Study the drawing (mm; zero at the part's minimum x, y, z) and answer. A direction names the side the tool comes from. Round coordinates to 2 decimals unless told otherwise and drop trailing zeros. Write each loop counter-clockwise with the first axis right and the second up, starting at its lowest first coordinate (ties: lowest second). Pieces come first, ordered by that corner, then holes. Notation, with made-up numbers: (19.5, -12.75) - (33.5, -12.75) arc R27 ccw to (33.5, 23.25) - close; hole circle Ø11 at (23, -26). An arc over 180 degrees is marked (long way). Use one line per item in the form item = value. Start each with the question number.
1) For a pull along Z with two mould halves and no side action, classify the marked faces 1, 2, 3 and 4 as released by +Z, released by -Z, zero draft, split by the parting line, or undercut.
2) Each of these flat-tipped pins is pushed along its axis until it touches: pin 1 (8.5 mm diameter, centred on y = 7, z = 6, fed in from +X); pin 2 (3 mm diameter, centred on x = 4.5, y = 5.5, fed in from -Z); pin 3 (3 mm diameter, centred on x = 3.5, y = 2.5, fed in from -Z); pin 4 (5 mm diameter, centred on x = 15, z = 37.5, fed in from -Y). Where does it stop, or does it pass through?
3) The part is cut by section D-D, the plane x = 15. Give the vertices of the cut face in (y, z) (3 decimals), plus the area to 3 significant figures.
4) Consider line 1 along X through (y, z) = (8.25, 12.35) (3 decimals); line 2 along Z through (x, y) = (1.25, 6.5); line 3 along Y through (x, z) = (8, 46). Determine where each line is inside the solid, lowest interval first. Write a range as from..to.
5) The part is cut by section A-A, the plane y = 7. Give the vertices of the cut face in (x, z) (3 decimals).
6) The part is cut by section B-B, the plane x = 10.25. Give the vertices of the cut face in (y, z) (3 decimals), plus the area to 3 significant figures.
7) The part is cut by section C-C, the plane z = 52. Give the vertices of the cut face in (x, y), plus the area to 3 significant figures.
8) For the marked faces 5, 6 and 7, determine the directions among +Z, -Z, +X, -X, +Y, -Y from which every point of the face is accessible in a straight line to the end or side of a thin tool.
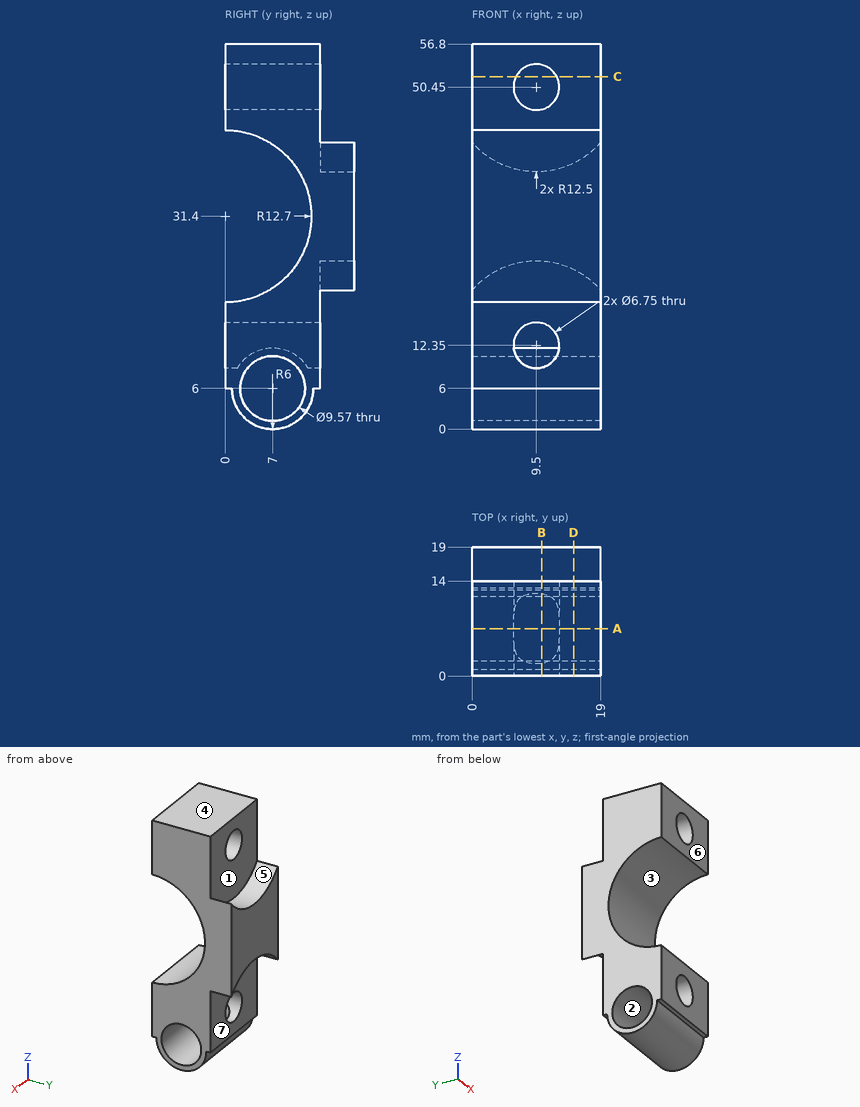
Geometry results:
q1.face_1 = zero draft
q1.face_2 = undercut
q1.face_3 = undercut
q1.face_4 = released by +Z
q2.pin_1 = through
q2.pin_2 = 0
q2.pin_3 = 0.8
q2.pin_4 = 9.35
q3.outline = (0, 6) - (1, 6) arc R6 ccw to (13, 6) - (14, 6) - (14, 23.575) - (19, 23.575) - (19, 39.225) - (14, 39.225) - (14, 56.8) - (0, 56.8) - (0, 44.1) arc R12.7 cw to (0, 18.7) - close; hole circle Ø9.57 at (7, 6)
q3.area = 521 mm2
q4.line_1 = 0..6.125, 12.875..19
q4.line_2 = 0.02..1.24, 10.76..20.49, 42.31..56.8
q4.line_3 = 0..14
q5.outline = (0, 0) - (19, 0) - (19, 1.215) - (0, 1.215) - close; (0, 10.785) - (19, 10.785) - (19, 20.803) - (0, 20.803) - close; (0, 41.997) - (19, 41.997) - (19, 56.8) - (0, 56.8) - close; hole circle Ø6.75 at (9.5, 50.45); hole (6.143, 12) - (12.857, 12) arc R3.375 ccw (long way) to start
q6.outline = (0, 6) - (1, 6) arc R6 ccw to (13, 6) - (14, 6) - (14, 9.059) - (12.161, 9.059) arc R6 ccw to (1.839, 9.059) - (0, 9.059) - close; (0, 15.641) - (14, 15.641) - (14, 24.827) - (19, 24.827) - (19, 37.973) - (14, 37.973) - (14, 47.159) - (0, 47.159) - (0, 44.1) arc R12.7 cw to (0, 18.7) - close; (0, 53.741) - (14, 53.741) - (14, 56.8) - (0, 56.8) - close; hole circle Ø9.57 at (7, 6)
q6.area = 345 mm2
q7.outline = (0, 0) - (6.5, 0) - (6.5, 14) - (0, 14) - close; (12.5, 0) - (19, 0) - (19, 14) - (12.5, 14) - close
q7.area = 182 mm2
q8.face_5 = +Z, +Y
q8.face_6 = +Z, -Z, +X, -X, -Y
q8.face_7 = -Z, +Y
